Work out the finished part from the listing and answer in its coordinate system (mm). A direction names the side the tool comes from. Give positions to 0.01 mm unless a question says otherwise; leave off trailing zeros. Write each loop counter-clockwise with the first axis right and the second up, starting at its lowest first coordinate (ties: lowest second). Pieces come first, ordered by that corner, then holes.
1) A tool of negligible diameter and unlimited length cuts with its end or side. For faces 1 (the face through (-0.541, 21.944, 14.793)), 2 (the face through (0, 15, -17)), from which of +Z, -Z, +X, -X, +Y, -Y can it reach the whole face along a straight path? Write none if from no direction.
2) Straight lines are drawn through the part: probe 1 along X at (y, z) = (13.75, -7.5); probe 2 along X at (y, z) = (6, -7); probe 3 along Z at (x, y) = (12, 12.5). For each, find the intervals that lie inside material, in ascending order.
3) Find section D-D (y = 17). Determine the outline of the cut face in (x, z) (3 decimals), plus the area to 3 significant figures.
4) Find section C-C (y = 6.25). Determine the outline of the cut face in (x, z) (3 decimals).
5) Find section B-B (z = 16.51). Determine the outline of the cut face in (x, y) (3 decimals).
6) Given pin 1 Ø5 at (x, y) = (-7.5, 19.5) entering from -Z; pin 2 Ø1.5 at (x, y) = (7, 12) entering from +Z; pin 3 Ø3 at (x, z) = (1, 16) entering from -Y; pin 4 Ø7.5 at (x, z) = (-14.3, -8.26) entering from -Y, each flat-ended and moving along its own axis, determine where each tip first touches the part or whether it passes through.
```python
from build123d import *
from OCP.BRepFilletAPI import BRepFilletAPI_MakeChamfer

# Parameters (mm, degrees)
SKETCH2_R                     = 27
BOSS_EXTRUDE2_DEPTH           = 26
CBORE_FOR_M3_SHCS1_AT_2_COUNT = 2
CBORE_FOR_M3_SHCS1_AT_2_PITCH = 28.596158833
CBORE_FOR_M3_SHCS1_AT_3_COUNT = 2
CBORE_FOR_M3_SHCS1_AT_3_PITCH = 28.596158833
HOLE1_D                       = 6.4
HOLE1_DEPTH                   = 15
HOLE1_CBORE_D                 = 7.3
HOLE1_CBORE_DEPTH             = 2
CHAMFER1_SIZE                 = 2
CHAMFER1_SIZE_2               = 0.45


with BuildPart() as part:
    # Sketch2 → Boss-Extrude2 (new body)
    with BuildSketch(Plane(origin=(0, 0, 0), x_dir=(1, 0, 0), z_dir=(0, 1, 0))):
        with Locations(Location((0, 0, 0), (0, 0, 90))):
            Circle(SKETCH2_R)
    extrude(amount=BOSS_EXTRUDE2_DEPTH)

    # Sketch5 → CBORE for M3 SHCS1 (revolve, cut)
    with BuildSketch(Plane(origin=(0, 0, 16.51), x_dir=(0, 0, -1), z_dir=(1, 0, 0))):
        Polygon((0, 0), (0, 26), (1.8, 26), (1.8, 18), (3.25, 18), (3.25, 0.025), (3.275, 0), align=None)
    cbore_for_m3_shcs1 = revolve(axis=Axis((0, -6.35, 16.51), (0, 1, 0)), mode=Mode.SUBTRACT)

    # CBORE for M3 SHCS1 at 2: CBORE for M3 SHCS1 ×2
    with Locations(*[Vector(0.5000000000000012, 0, -0.8660254037844379) * (i * CBORE_FOR_M3_SHCS1_AT_2_PITCH) for i in range(1, CBORE_FOR_M3_SHCS1_AT_2_COUNT)]):
        add(cbore_for_m3_shcs1, mode=Mode.SUBTRACT)

    # CBORE for M3 SHCS1 at 3: CBORE for M3 SHCS1 ×2
    with Locations(*[Vector(-0.4999999999999978, 0, -0.8660254037844399) * (i * CBORE_FOR_M3_SHCS1_AT_3_PITCH) for i in range(1, CBORE_FOR_M3_SHCS1_AT_3_COUNT)]):
        add(cbore_for_m3_shcs1, mode=Mode.SUBTRACT)

    # Hole1
    with Locations(Plane(origin=(0, 0, 0), x_dir=(-1, 0, 0), z_dir=(0, -1, 0))):
        with Locations((14.298079416, -8.255), (0, 16.51), (-14.298079416, -8.255)):
            CounterBoreHole(HOLE1_D / 2, HOLE1_CBORE_D / 2, HOLE1_CBORE_DEPTH, depth=HOLE1_DEPTH)

    # Chamfer1
    chamfer1_edges_1 = [part.edges().sort_by_distance(p)[0] for p in [
        (17.948079416, 2, 8.255),
    ]]
    chamfer1_side_1 = [part.faces().sort_by_distance(p)[0] for p in [
        (17.948079416, 1.991, 8.255),
    ]]
    chamfer1_edges_2 = [part.edges().sort_by_distance(p)[0] for p in [
        (3.65, 2, -16.51),
    ]]
    chamfer1_side_2 = [part.faces().sort_by_distance(p)[0] for p in [
        (3.65, 1.991, -16.51),
    ]]
    chamfer1_edges_3 = [part.edges().sort_by_distance(p)[0] for p in [
        (-10.648079416, 2, 8.255),
    ]]
    chamfer1_side_3 = [part.faces().sort_by_distance(p)[0] for p in [
        (-10.648079416, 1.991, 8.255),
    ]]
    chamfer1 = BRepFilletAPI_MakeChamfer(part.part.solid().wrapped)
    for e in chamfer1_edges_1:
        chamfer1.Add(CHAMFER1_SIZE - 0.0001, CHAMFER1_SIZE_2 - 0.0001, e.wrapped, chamfer1_side_1[0].wrapped)
    for e in chamfer1_edges_2:
        chamfer1.Add(CHAMFER1_SIZE - 0.0001, CHAMFER1_SIZE_2 - 0.0001, e.wrapped, chamfer1_side_2[0].wrapped)
    for e in chamfer1_edges_3:
        chamfer1.Add(CHAMFER1_SIZE - 0.0001, CHAMFER1_SIZE_2 - 0.0001, e.wrapped, chamfer1_side_3[0].wrapped)
    add(Compound.cast(chamfer1.Shape()), mode=Mode.REPLACE)  # a hair under: the kernel refuses the full size


solid = part.part
```
Results:
1. face 1: +Y, -Y
1. face 2: -Y
2. probe 1: x = -25.94 to -17.46, -11.14 to 11.14, 17.46 to 25.94
2. probe 2: x = -26.08 to -17.3, -11.3 to 11.3, 17.3 to 26.08
2. probe 3: z = -24.19 to -10.55, -5.96 to 6.03, 10.48 to 24.19
3. outline: circle Ø54 at (0, 0); hole circle Ø6.5 at (-14.298, -8.255); hole circle Ø6.5 at (0, 16.51); hole circle Ø6.5 at (14.298, -8.255)
3. area: 2,190 mm2
4. outline: circle Ø54 at (0, 0); hole circle Ø6.5 at (-14.298, -8.255); hole circle Ø6.4 at (-14.298, 8.255); hole circle Ø6.5 at (0, 16.51); hole circle Ø6.4 at (0, -16.51); hole circle Ø6.5 at (14.298, -8.255); hole circle Ø6.4 at (14.298, 8.255)
5. outline: (-21.364, 0) - (-3.275, 0) - (-3.25, 0.025) - (-3.25, 18) - (-1.8, 18) - (-1.8, 26) - (-21.364, 26) - close; (1.8, 18) - (3.25, 18) - (3.25, 0.025) - (3.275, 0) - (21.364, 0) - (21.364, 26) - (1.8, 26) - close
6. pin 1: stops at z = -26.53
6. pin 2: stops at z = 26.27
6. pin 3: stops at y = 18
6. pin 4: stops at y = 0
